Check sheet for the modelled part. Datum: model origin and axes. Units: mm. A direction names the side the tool comes from. Give positions to 0.01 mm unless a question says otherwise; leave off trailing zeros. Loops run counter-clockwise (first coordinate to the right, second up) from the corner with the lowest first, then second, coordinate; pieces in that order, holes last. Notation, with made-up numbers: (66.5, 89) - (89.5, 89) arc R36 ccw to (89.5, 125) - close; hole circle Ø4 at (45.5, -2.75). An arc over 180 degrees is marked (long way). Use CSV: the item, a comma, the result in double quotes.
Autodesk Inventor part; units mm, degrees
ref_plane "YZ Plane" through (0, 0, 0) normal (1, 0, 0) x (0, 1, 0)
ref_plane "XZ Plane" through (0, 0, 0) normal (0, 1, 0) x (-1, 0, 0)
ref_plane "XY Plane" through (0, 0, 0) normal (0, 0, 1) x (1, 0, 0)
sketch "Sketch1" plane through (0, 0, 0) normal (0, 0, 1) x (1, 0, 0)
  line L0 (-26.36, -35.13) -> (26.36, -35.13)
  line L1 (26.36, -35.13) -> (26.36, 35.13)
  line L2 (26.36, 35.13) -> (-26.36, 35.13)
  line L3 (-26.36, 35.13) -> (-26.36, -35.13)
  line L4 (-26.36, -35.13) -> (26.36, 35.13) construction
  line L5 (26.36, -35.13) -> (-26.36, 35.13) construction
  line L6 (-21.36, -30.13) -> (21.36, -30.13)
  line L7 (21.36, -30.13) -> (21.36, 30.13)
  line L8 (21.36, 30.13) -> (-21.36, 30.13)
  line L9 (-21.36, 30.13) -> (-21.36, -30.13)
  line L10 (-21.36, -30.13) -> (21.36, 30.13) construction
  line L11 (21.36, -30.13) -> (-21.36, 30.13) construction
  point P0 (0, 0)
  dimension "t" = 5
  dimension "d1" = 5
  dimension "d2" = 60.26
  dimension "d3" = 42.72
extrude "Extrusion1" add sketch "Sketch1" along normal blind 3.2
sketch "Sketch2" plane through (0, 0, 3.2) normal (0, 0, 1) x (1, 0, 0)
  line L0 (-11.5572, -30.63) -> (-3.5572, -30.63)
  arc A0 (-3.5572, -30.63) -> (-2.7846, -30.4157) centre (-3.5572, -29.13) ccw
  arc A1 (-1.7544, -30.13) -> (-2.7846, -30.4157) centre (-1.7544, -32.13) ccw
  line L1 (21.36, -30.13) -> (-21.36, -30.13)
  line L2 (-7.5572, -30.63) -> (-7.5572, -30.13)
  arc A2 (-12.3298, -30.4157) -> (-11.5572, -30.63) centre (-11.5572, -29.13) ccw
  arc A3 (-12.3298, -30.4157) -> (-13.36, -30.13) centre (-13.36, -32.13) ccw
  point P0 (0, 0)
  point P1 (-13.36, -30.13)
  dimension "d6" = 0.5
  dimension "d7" = 8
  dimension "d8" = 1.5
  dimension "d9" = 2
  dimension "d10" = 8
extrude "Extrusion2" cut sketch "Sketch2" against normal blind 3.2
equation "\"d1\" = t"
properties part number "LCDFrame"
1. Sectioned sample at C-C, the plane z = 1.9. Record the boundary of the cut face in (x, y), and give its area (3 significant figures).
Completed:
outline,"(-26.36, -35.13) - (26.36, -35.13) - (26.36, 35.13) - (-26.36, 35.13) - close; hole (-21.36, -30.13) - (-13.36, -30.13) arc R2 cw to (-12.33, -30.42) arc R1.5 ccw to (-11.56, -30.63) - (-3.56, -30.63) arc R1.5 ccw to (-2.78, -30.42) arc R2 cw to (-1.75, -30.13) - (21.36, -30.13) - (21.36, 30.13) - (-21.36, 30.13) - close"
area,"1,120 mm²"
2. Release check for a two-part mould opening along X. For faces 1 (the face through (-26.36, 0, 2)), 2 (the face through (26.36, 0, 2)), 3 (the face through (0, 30.13, 2)) record: released by +X, released by -X, zero draft, split by the parting line, or undercut.
Completed:
face 1,"released by -X"
face 2,"released by +X"
face 3,"undercut"
3. Sectioned sample at B-B, the plane y = 5. Record the boundary of the cut face in (x, z), and give its area (3 significant figures).
Completed:
outline,"(-26.36, 0) - (-21.36, 0) - (-21.36, 3.2) - (-26.36, 3.2) - close; (21.36, 0) - (26.36, 0) - (26.36, 3.2) - (21.36, 3.2) - close"
area,"32.0 mm²"
4. Set-up check for faces 4 (the face through (0, 35.13, 2)), 5 (the face through (-17, -30.13, 2)): record each of +Z, -Z, +X, -X, +Y, -Y from which the full face is reachable in a straight line by a thin tool's end or side.
Completed:
face 4,"+Z, -Z, +X, -X, +Y"
face 5,"+Z, -Z"
5. Sectioned sample at A-A, the plane x = -10.5. Record the boundary of the cut face in (y, z).
Completed:
outline,"(-35.13, 0) - (-30.63, 0) - (-30.63, 3.2) - (-35.13, 3.2) - close; (30.13, 0) - (35.13, 0) - (35.13, 3.2) - (30.13, 3.2) - close"
6. Scan lines: line 1 along Y through (x, z) = (-9.5, 0.6); line 2 along Y through (x, z) = (9.5, 1.5); line 3 along X through (y, z) = (28, 0.6). Record each from-to range of solid material in increasing order.
Completed:
line 1,"y = -35.13 to -30.63, 30.13 to 35.13"
line 2,"y = -35.13 to -30.13, 30.13 to 35.13"
line 3,"x = -26.36 to -21.36, 21.36 to 26.36"
